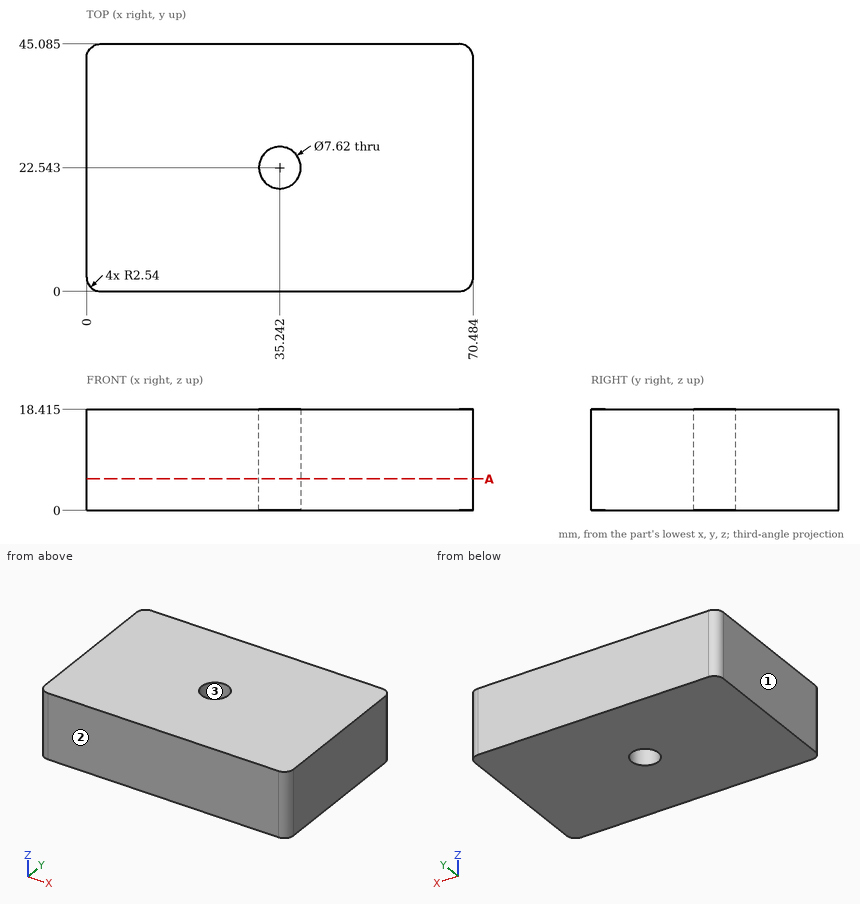
For this review, use the dimensioned drawing (mm, ordinates from the lowest corner) and the shaded views. Coordinates: 2 decimals unless noted, no trailing zeros. Order: outer loops, then holes, each group sorted by start corner. A loop starts at its lowest first (then second) coordinate and runs counter-clockwise, first axis right, second up. Notation, with made-up numbers: (81, -14.5) - (88, -14.5) arc R27 ccw to (88, 6.5) - close; hole circle Ø1 at (-31, -32.5). An arc over 180 degrees is marked (long way). Use one line per item in the form item = value.
Q1. For P1, Ø12, axis at x = 39.5, y = 13.5, coming from the -Z side; P2, Ø6, axis at x = 35.24, y = 22.54, coming from the -Z side, all flat-tipped, find the tip position at first contact; note any pin that passes through.
Checked values:
P1 = 0
P2 = through
Q2. Draft analysis for pull direction X (two halves, no side actions). For the marked faces 1, 2 and 3, state which applies: +X half, -X half, draft (parallel to the pull), parting line (faces both ways), or undercut.
Checked values:
face_1 = -X half
face_2 = draft
face_3 = undercut
Q3. For probe 1 along X at (y, z) = (43, 9); probe 2 along X at (y, z) = (2, 12.5) (1 decimal), list the stretches that pass through material, from the lowest coordinate up. Write a range as from..to.
Checked values:
probe_1 = 0.04..70.44
probe_2 = 0.1..70.4
Q4. Consider section A-A (z = 5.75). Give the boundary of the cut face in (x, y) (1 decimal).
Checked values:
outline = (0, 2.5) arc R2.5 ccw to (2.5, 0) - (67.9, 0) arc R2.5 ccw to (70.5, 2.5) - (70.5, 42.5) arc R2.5 ccw to (67.9, 45.1) - (2.5, 45.1) arc R2.5 ccw to (0, 42.5) - close; hole circle Ø7.6 at (35.2, 22.5)
